Study the drawing (mm; zero at the part's minimum x, y, z) and answer. Give positions to 0.01 mm unless a question says otherwise; leave off trailing zeros. Write each loop counter-clockwise with the first axis right and the second up, starting at its lowest first coordinate (ties: lowest second). Pieces come first, ordered by that corner, then holes. Notation, with made-up numbers: (-10, 9) - (10, 9) arc R28 cw to (10, 39) - close; hole circle Ø9 at (24.5, 46). An arc over 180 degrees is marked (long way). One line per item, written item: value. Start each with the question number.
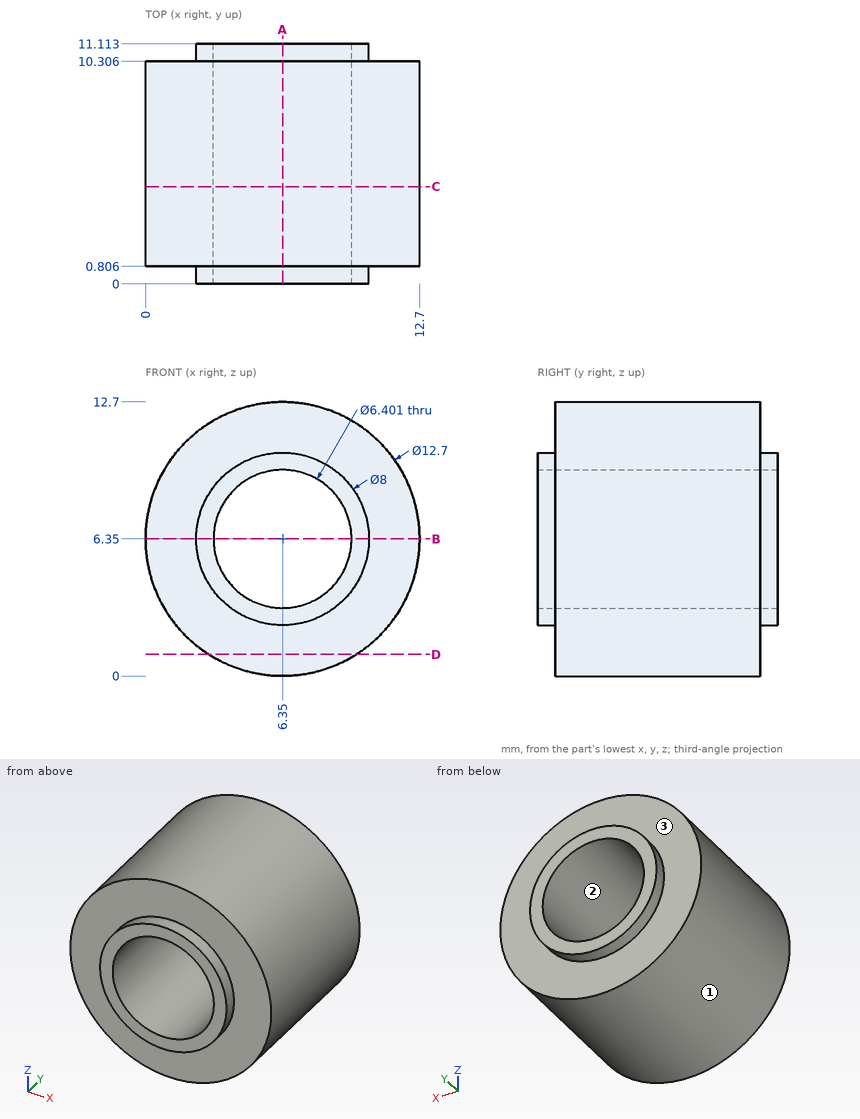
Item 1: Find section D-D on z = 1. Determine the outline of the cut face in (x, y).
Item 2: Find section B-B on z = 6.35. Determine the outline of the cut face in (x, y).
Item 3: The mould has two halves that part along X. Classify the marked faces 1, 2 and 3: +X half, -X half, draft (parallel to the pull), parting line (faces both ways), or undercut.
Item 4: Each of these flat-tipped pins is pushed along its axis until it touches: pin 1 Ø5 at (y, z) = (5.5, 10.5) entering from +X; pin 2 Ø2 at (y, z) = (6.5, 4) entering from +X (1 decimal); pin 3 Ø4 at (x, y) = (11, 1) entering from +Z. Where does it stop, or does it pass through?
Item 5: Straight lines are drawn through the part: line 1 along X through (y, z) = (7.75, 6.25); line 2 along Y through (x, z) = (1.5, 3.5). For each, find the intervals that lie inside material, in ascending order.
Item 6: Find section C-C on y = 4.5. Determine the outline of the cut face in (x, z).
Item 7: Find section A-A on x = 6.35. Determine the outline of the cut face in (y, z).
Values:
1. outline: (2.93, 0.81) - (9.77, 0.81) - (9.77, 10.31) - (2.93, 10.31) - close
2. outline: (0, 0.81) - (2.35, 0.81) - (2.35, 0) - (3.15, 0) - (3.15, 11.11) - (2.35, 11.11) - (2.35, 10.31) - (0, 10.31) - close; (9.55, 0) - (10.35, 0) - (10.35, 0.81) - (12.7, 0.81) - (12.7, 10.31) - (10.35, 10.31) - (10.35, 11.11) - (9.55, 11.11) - close
3. face 1: parting line
3. face 2: undercut
3. face 3: draft
4. pin 1: x = 12.48
4. pin 2: x = 12.6
4. pin 3: z = 12.12
5. line 1: 0 to 3.15, 9.55 to 12.7
5. line 2: 0.81 to 10.31
6. outline: circle Ø12.7 at (6.35, 6.35); hole circle Ø6.4 at (6.35, 6.35)
7. outline: (0, 2.35) - (0.81, 2.35) - (0.81, 0) - (10.31, 0) - (10.31, 2.35) - (11.11, 2.35) - (11.11, 3.15) - (0, 3.15) - close; (0, 9.55) - (11.11, 9.55) - (11.11, 10.35) - (10.31, 10.35) - (10.31, 12.7) - (0.81, 12.7) - (0.81, 10.35) - (0, 10.35) - close
